Verification items for the finished model (mm, model axes). A direction names the side the tool comes from. Round coordinates to 2 decimals unless told otherwise and drop trailing zeros. Order: outer loops, then holes, each group sorted by start corner. A loop starts at its lowest first (then second) coordinate and runs counter-clockwise, first axis right, second up. Notation, with made-up numbers: M 43.25,83.5 L 80.25,83.5 A28 ccw 80.25,112.5 Z; hole C -33,32.5 d4. An arc over 180 degrees is marked long. One line per item, written item: value. Start each with the question number.
from build123d import *

# Parameters (mm, degrees)
F0_W     = 330.2
F0_H     = 12.7
F0_R     = 2.032
F1_DEPTH = 6.35
F2_R     = 2.54
F3_W     = 8.6677474901
F3_H     = 8.4455003962
F4_DEPTH = 330.2


with BuildPart() as f1:
    # F0 (on Front) → F1 (new body, symmetric)
    with BuildSketch(Plane.XZ):
        Rectangle(F0_W, F0_H)
        with Locations((-154.94, 0)):
            Circle(F0_R, mode=Mode.SUBTRACT)
        Circle(F0_R, mode=Mode.SUBTRACT)
        with Locations((154.94, 0)):
            Circle(F0_R, mode=Mode.SUBTRACT)
    extrude(amount=F1_DEPTH, both=True)

    # F2
    f2_edges = [f1.edges().sort_by_distance(p)[0] for p in [
        (165.1, 0, -6.35),
        (165.1, 6.35, 0),
        (165.1, -6.35, 0),
    ]]
    fillet(f2_edges, radius=F2_R)

    # F3 (on face) → F4 (cut)
    with BuildSketch(Plane(origin=(-165.1, 0, 0), x_dir=(0, -1, 0), z_dir=(-1, 0, 0))):
        Rectangle(F3_W, F3_H)
    extrude(amount=-F4_DEPTH, mode=Mode.SUBTRACT)


solid = f1.part
1. Tool access check on faces 1 (the face through (-2, 0, 6.35)), 2 (the face through (-2.3, 4.334, -0.1)). Record the directions out of +Z, -Z, +X, -X, +Y, -Y that give a thin tool (end or side, any length) a straight path to the whole face; none if there is none.
2. Depth check by flat-ended pin: pin 1 (3.5 mm diameter, centred on x = 0, z = 0, fed in from +Y). Enter the tip coordinate at first touch or a pass-through.
3. Scan lines: line 1 along Y through (x, z) = (-27, 1.75); line 2 along X through (y, z) = (-5.45, 0); line 3 along Z through (x, y) = (-136, -3.25). Record each from-to range of solid material in increasing order.
4. Section check C-C (x = 94). Record the cut outline in (y, z), and give its area (3 significant figures).
5. Section check A-A (z = 0). Give the number of separate pieces and of enclosed holes in the cut face, and give its area (3 significant figures).
6. Section check B-B (y = -1.5). Record the cut outline in (x, z).
Geometry check:
1. face 1: +Z, +X, -X, +Y, -Y
1. face 2: +X, -X
2. pin 1: passes through
3. line 1: y = -6.35 to -4.33, 4.33 to 6.35
3. line 2: x = -165.1 to -156.97, -152.91 to -2.03, 2.03 to 152.91, 156.97 to 164.5
3. line 3: z = -6.35 to -4.22, 4.22 to 6.35
4. outline: M -6.35,-6.35 L 6.35,-6.35 L 6.35,6.35 L -6.35,6.35 Z; hole M -4.33,-4.22 L 4.33,-4.22 L 4.33,4.22 L -4.33,4.22 Z
4. area: 88.1 mm²
5. separate pieces: 8
5. enclosed holes: 0
5. area: 1,280 mm²
6. outline: M -165.1,-6.35 L 162.56,-6.35 A2.54 ccw 165.07,-4.22 L -165.1,-4.22 Z; M -165.1,4.22 L 165.1,4.22 L 165.1,6.35 L -165.1,6.35 Z
